The listing builds one solid part. Answer for the finished solid, in the listing's coordinates (mm). A direction names the side the tool comes from. Coordinates: 2 decimals unless noted, no trailing zeros. Order: outer loops, then holes, each group sorted by start corner. A loop starts at its lowest first (then second) coordinate and runs counter-clockwise, first axis right, second up. Notation, with made-up numbers: (53, 85) -> (58, 85) arc R15 ccw to (58, 104) -> close; hole circle Ø10 at (-31.5, 10.25). An arc over 180 degrees is marked (long way). Write each question's results on one line, items separated by ' | '. Start each with the question number.
(1) Given pin 1 (12 mm diameter, centred on x = 33, y = 151.5, fed in from +Z); pin 2 (6 mm diameter, centred on x = -48.5, y = 145.5, fed in from -Z); pin 3 (22 mm diameter, centred on y = 139, z = 22, fed in from +X), each flat-ended and moving along its own axis, determine where each tip first touches the part or whether it passes through.
(2) Straight lines are drawn through the part: L1, parallel to Y at x = 14, z = 48; L2, parallel to Y at x = -45, z = 29.5; L3, parallel to X at y = 97.5, z = -41. For each, find the intervals that lie inside material, in ascending order.
(3) A tool of negligible diameter and unlimited length cuts with its end or side. For faces 1 (the face through (60, 87, -9)), 2 (the face through (-40, 140, 25)), 3 (the face through (-1, 62, 40)), 4 (the face through (100, 57.541, -82)), 5 (the face through (-1, 60, -60)), from which of +Z, -Z, +X, -X, +Y, -Y can it reach the whole face along a straight path? Write none if from no direction.
(4) The part is cut by section C-C, the plane y = 63.5. Give the vertices of the cut face in (x, z).
(5) The part is cut by section A-A, the plane x = -26.5. Give the vertices of the cut face in (y, z), then the cut area to 4 significant figures.
(6) The part is cut by section B-B, the plane z = -4.5. Give the vertices of the cut face in (x, y).
(7) Determine the mould class of faces 6 (the face through (-50, 146, 17.607)), 7 (the face through (-1, 11, 43)), 8 (the face through (-100, 5, 1)) for opening direction X: +X half, -X half, draft (parallel to the pull), parting line (faces both ways), or undercut.
(8) The part is cut by section D-D, the plane y = 121. Give the vertices of the cut face in (x, z).
Autodesk Inventor part; units mm, degrees
ref_plane "Work Plane1" through (90, 11, -90) normal (1, 0, 0) x (0, 1, 0)
sketch "Sketch1" plane through (0, 0, 0) normal (1, 0, 0) x (0, 1, 0)
  line L0 (11, 100) -> (0, 100)
  line L1 (0, 100) -> (0, -100)
  line L2 (0, -100) -> (11, -100)
  line L3 (11, -100) -> (11, 100)
  line L4 (-2.2, 0) -> (13.2, 0)
  line L5 (0, 140) -> (0, -140)
  point P0 (0, 0)
  point P1 (11, 0)
  dimension "d0" = 200
  dimension "d1" = 11
  dimension "d2" = 0
extrude "Extrusion1" add sketch "Sketch1" along normal mid plane 200
sketch "Sketch2" plane through (0, 0, 0) normal (1, 0, 0) x (0, 1, 0)
  line L0 (111, 40) -> (11, 40)
  line L1 (11, 40) -> (11, -60)
  line L2 (11, -60) -> (111, -60)
  line L3 (111, -60) -> (111, 40)
  line L4 (-32.1032, 0) -> (192.619, 0)
  line L5 (11, -100) -> (11, 100)
  line L6 (111, 40) -> (161, 40)
  line L7 (161, 40) -> (161, -10)
  line L8 (161, -10) -> (111, -10)
  line L9 (111, -10) -> (111, 40)
  line L10 (111, -60) -> (211, -60)
  line L11 (211, -60) -> (211, -10)
  line L12 (211, -10) -> (111, -10)
  line L13 (111, -10) -> (111, -60)
  line L14 (111, 40) -> (161, -10)
  line L15 (111, -60) -> (211, -10)
  point P0 (0, 0)
  dimension "d5" = 100
  dimension "d6" = 40
  dimension "d7" = 100
  dimension "d8" = 0
  dimension "d9" = 50
  dimension "d10" = 50
  dimension "d11" = 100
  dimension "d12" = 50
extrude "Extrusion2" add sketch "Sketch2" along normal mid plane 120 contours L3 L4 L1 L0 | L14 L4 L3 | L4 L14 L8 L3 | L3 L2 L1 L4 | L8 L12 L15 L3
sketch "Sketch3" plane through (-60, 0, 0) normal (-1, 0, 0) x (0, 0, 1)
  line L0 (15.607, 155.393) -> (35.607, 155.393)
  line L1 (35.607, 155.393) -> (35.607, 135.393)
  line L2 (35.607, 135.393) -> (15.607, 135.393)
  line L3 (15.607, 135.393) -> (15.607, 155.393)
  line L4 (40, 111) -> (-10, 161)
  line L5 (35.607, 135.393) -> (35.607, 115.393)
  line L6 (-10, 161) -> (40, 111)
  line L7 (15.607, 135.393) -> (35.607, 115.393)
  point P0 (0, 0)
  dimension "d15" = 20
  dimension "d16" = 20
  dimension "d17" = 4.393
extrude "Extrusion3" add sketch "Sketch3" against normal blind 20
sketch "Sketch4" plane through (-60, 155.393, 35.607) normal (0, 1, 0) x (1, 0, 0)
  line L0 (20, 20) -> (20, 0)
  line L1 (0, 20) -> (20, 20)
  line L2 (0, 0) -> (0, 20)
  line L3 (0, 0) -> (20, 0)
  line L4 (18, 2) -> (18, 18)
  line L5 (18, 18) -> (2, 18)
  line L6 (2, 18) -> (2, 2)
  line L7 (2, 2) -> (18, 2)
  point P0 (60, 35.607)
  dimension "d20" = 2
extrude "Extrusion4" cut sketch "Sketch4" against normal blind 20 contours L7 L6 L5 L4
sketch "Sketch5" plane through (-100, 11, 100) normal (0, 1, 0) x (1, 0, 0)
  line L0 (200, 200) -> (200, 0)
  line L1 (0, 200) -> (200, 200)
  point P0 (100, 100)
  point P1 (190, 190)
  dimension "d23" = 10
  dimension "d24" = 10
ref_plane "Work Plane1" through (90, 11, -90) normal (1, 0, 0) x (0, 1, 0)
sketch "Sketch7" plane through (90, 11, -90) normal (1, 0, 0) x (0, 1, 0)
  line L0 (0, -10) -> (0, 190)
  line L1 (0, 0) -> (20, 0)
  line L2 (20, 0) -> (20, 5)
  line L3 (20, 5) -> (0, 5)
  line L4 (0, 5) -> (0, 0)
  line L5 (20, 0) -> (20, 20)
  line L6 (90, 0) -> (60.481, 11.7284)
  line L7 (60.481, 11.7284) -> (60.481, 5)
  line L8 (60.481, 9.4368) -> (46.541, 14.9754)
  line L9 (46.541, 14.9754) -> (46.541, 5)
  line L10 (46.541, 12.5046) -> (32.601, 18.0432)
  line L11 (32.601, 18.0432) -> (32.601, 5)
  line L12 (32.601, 15.2739) -> (20, 20)
  line L13 (90, 0) -> (20, 0)
  point P0 (-11, 90)
  dimension "d25" = 20
  dimension "d26" = 5
  dimension "d27" = 20
  dimension "d28" = 15
  dimension "d29" = 15
revolve "Revolution1" add sketch "Sketch7" angle 360 about axis through (90, 101, -90) along (0, -1, 0)
properties part number "House_Assembly_Depth_Tracking"
Established:
1) pin 1: stops at z = 5.5 | pin 2: stops at z = -44.25 | pin 3: stops at x = 60
2) L1: y = 0 to 11 | L2: y = 0 to 135.39 | L3: x = -60 to 60
3) face 1: +Z, -Z, +X, +Y | face 2: +Z, +X, +Y | face 3: +Z, +X, -X, +Y | face 4: none | face 5: -Z, +X, -X, +Y
4) outline: (-60, -60) -> (60, -60) -> (60, 40) -> (-60, 40) -> close; circle Ø25.22 at (90, -90)
5) outline: (0, -100) -> (11, -100) -> (11, -60) -> (111, -60) -> (211, -10) -> (161, -10) -> (111, 40) -> (11, 40) -> (11, 100) -> (0, 100) -> close | area: 15,950 mm^2
6) outline: (-100, 0) -> (100, 0) -> (100, 11) -> (60, 11) -> (60, 155.5) -> (-60, 155.5) -> (-60, 11) -> (-100, 11) -> close
7) face 6: undercut | face 7: draft | face 8: -X half
8) outline: (-60, -55) -> (60, -55) -> (60, 30) -> (-40, 30) -> (-40, 35.61) -> (-60, 35.61) -> close
